Can you work these out from the model? Positions are in its coordinate system, mm. A direction names the side the tool comes from. Give positions to 0.01 mm unless a question says otherwise; leave off trailing zeros. Order: outer loops, then holes, each group sorted by start corner. A loop starts at its lowest first (then second) coordinate and runs counter-clockwise, first axis right, second up. Notation, with made-up numbers: M 67.5,-9 L 107.5,-9 A3 ccw 107.5,-4 Z; hole C -4,-38 d4. An arc over 180 degrees is marked long. Answer as a JSON object with one key per item and string values.
```python
from build123d import *

# Parameters (mm, degrees)
SKETCH2_R           = 9
BOSS_EXTRUDE1_DEPTH = 40
CUT_EXTRUDE1_DEPTH  = 10
FILLET1_R           = 1
FILLET2_R           = 1


with BuildPart() as part:
    # Sketch2 → Boss-Extrude1 (new body)
    with BuildSketch(Plane(origin=(0, 0, 0), x_dir=(1, 0, 0), z_dir=(0, 1, 0))):
        with Locations(Location((0, 0, 0), (0, 0, 270))):
            Circle(SKETCH2_R)
    extrude(amount=BOSS_EXTRUDE1_DEPTH)

    # Sketch4 → Cut-Extrude1 (cut)
    with BuildSketch(Plane.XZ):
        with BuildLine():
            Line((-2.867677405, 0.881150554), (2.867677405, 0.881150554))
            ThreePointArc((2.867677405, 0.881150554), (0, -3), (-2.867677405, 0.881150554))
        make_face()
    extrude(amount=-CUT_EXTRUDE1_DEPTH, mode=Mode.SUBTRACT)

    # Fillet1
    fillet1_edges = [part.edges().sort_by_distance(p)[0] for p in [
        (0, 0, -9),
    ]]
    fillet(fillet1_edges, radius=FILLET1_R)

    # Fillet2
    fillet2_edges = [part.edges().sort_by_distance(p)[0] for p in [
        (0, 40, -9),
    ]]
    fillet(fillet2_edges, radius=FILLET2_R)


solid = part.part
```
1) I want a section at B-B on z = 0. Write out the boundary of the cut face in (x, y).
Results found:
{"outline": "M -9,1 A1 ccw -8,0 L -3,0 L -3,10 L 3,10 L 3,0 L 8,0 A1 ccw 9,1 L 9,39 A1 ccw 8,40 L -8,40 A1 ccw -9,39 Z"}
2) I need wall thicknesses on L1, parallel to X at y = 7.5, z = 0; L2, parallel to Y at x = -6.5, z = -6; L3, parallel to Z at x = -7.25, y = 29. Which ranges of each line are inside material? Lowest first, please.
Results found:
{"L1": "x = -9 to -3, 3 to 9", "L2": "y = 0.47 to 39.53", "L3": "z = -5.33 to 5.33"}
3) Thinking about a two-plate mould opening in Z: for faces 1 (the face through (2.703, 19.734, 8.584)), 2 (the face through (0, 5, -3)), 3 (the face through (0, 0, 2)), which applies, pulls with the +Z half, pulls with the -Z half, needs draft (parallel to the pull), parting line crosses it, or undercut?
Results found:
{"face 1": "parting line crosses it", "face 2": "undercut", "face 3": "needs draft"}
4) I want a section at C-C on y = 27.5. Write out the boundary of the cut face in (x, z).
Results found:
{"outline": "C 0,0 d18"}
5) For faces 4 (the face through (0, 40, 0)), 5 (the face through (0, 5, 0.881)), which set-ups out of +Z, -Z, +X, -X, +Y, -Y let a thin tool reach every point of the face, with its end or its side?
Results found:
{"face 4": "+Z, -Z, +X, -X, +Y", "face 5": "-Y"}
6) I'm going to push flat-ended pins straight in: pin 1 Ø1.5 at (x, y) = (-7, 17.5) entering from +Z; pin 2 Ø3 at (y, z) = (7.5, 7) entering from +X; pin 3 Ø3 at (y, z) = (8.5, 2) entering from +X. Where does each tip first touch, or does it pass through?
Results found:
{"pin 1": "stops at z = 6.48", "pin 2": "stops at x = 7.12", "pin 3": "stops at x = 8.99"}
7) I want a section at A-A on x = 0. Write out the boundary of the cut face in (y, z), and give its area (3 significant figures).
Results found:
{"outline": "M 0,-8 A1 ccw 1,-9 L 39,-9 A1 ccw 40,-8 L 40,8 A1 ccw 39,9 L 1,9 A1 ccw 0,8 L 0,0.88 L 10,0.88 L 10,-3 L 0,-3 Z", "area": "680 mm²"}
